```python
from build123d import *

# Parameters (mm, degrees)
PAD_DEPTH = 20
FILLET_R  = 2


with BuildPart() as part:
    # Sketch → Pad (new body)
    with BuildSketch(Plane.XZ):
        Polygon((0, 0), (18, 0), (16.5, 10), (1.5, 10), align=None)
    extrude(amount=PAD_DEPTH)

    # Fillet
    fillet_edges = [part.edges().sort_by_distance(p)[0] for p in [
        (0.75, 0, 5),
        (0.75, -20, 5),
        (17.25, -20, 5),
        (17.25, 0, 5),
    ]]
    fillet(fillet_edges, radius=FILLET_R)


solid = part.part
```
Verification items for the finished model (mm, model axes). Coordinates: 2 decimals unless noted, no trailing zeros. Write each loop counter-clockwise with the first axis right and the second up, starting at its lowest first coordinate (ties: lowest second). Pieces come first, ordered by that corner, then holes. Notation, with made-up numbers: M 45,-1 L 55,-1 A15 ccw 55,16 Z; hole C 27.5,-1.75 d5. An arc over 180 degrees is marked long. Answer as a JSON object with one key per item and string values. Group by question number.
(1) Cross-section at A-A, the plane y = -17. Record the cut outline in (x, z).
(2) Gauge pin test, flat ends, axial feed: pin 1 (4 mm diameter, centred on y = -9.5, z = 7.5, fed in from -X) (3 decimals); pin 2 (1.5 mm diameter, centred on y = -10.5, z = 4.5, fed in from +X); pin 3 (4 mm diameter, centred on y = -12, z = 4.5, fed in from -X) (3 decimals). Record the tip position at first contact, or that the pin passes through.
(3) Material ranges on line 1 (Y direction, x = 2, z = 3.5); line 2 (X direction, y = -5, z = 4.5) (3 decimals); line 3 (X direction, y = -16.75, z = 2.5) (3 decimals), recorded low to high.
(4) Release check for a two-part mould opening along Z. For faces 1 (the face through (9, -10, 0)), 2 (the face through (9, 0, 5)), 3 (the face through (1.325, -19.399, 4.992)) record: +Z half, -Z half, draft (parallel to the pull), parting line (faces both ways), or undercut.
Reply:
{
 "1": {"outline": "M 0,0 L 18,0 L 16.5,10 L 1.5,10 Z"},
 "2": {"pin 1": "x = 0.825", "pin 2": "x = 17.44", "pin 3": "x = 0.375"},
 "3": {"line 1": "-19.93 to -0.07", "line 2": "0.675 to 17.325", "line 3": "0.375 to 17.625"},
 "4": {"face 1": "-Z half", "face 2": "draft", "face 3": "+Z half"}
}
